from build123d import *

# Parameters (mm, degrees)
SKETCH_2_W          = 58
SKETCH_2_H          = 22
EXTRUDE_1_DEPTH     = 5
SKETCH_4_R          = 10.25
SKETCH_4_R_2        = 1.8
CUT_EXTRUDE_1_DEPTH = 0.5
SKETCH_4_3_R        = 1.8
CUT_EXTRUDE_2_DEPTH = 10
SKETCH_5_W          = 35
SKETCH_5_H          = 4
CUT_EXTRUDE_3_DEPTH = 10
SKETCH_6_R          = 5
CUT_EXTRUDE_4_DEPTH = 3.5
CHAMFER_1_SIZE      = 0.5
CHAMFER_1_SIZE2     = 0.181985117
SKETCH_7_R          = 2
CUT_EXTRUDE_5_DEPTH = 3.5
FILLET_2_R          = 10
FILLET_3_R          = 6
FILLET_4_R          = 20
FILLET_5_R          = 7


with BuildPart() as part:
    # Эскиз2 → Бобышка-Вытянуть1 (new body)
    with BuildSketch(Plane(origin=(0, 0, 0), x_dir=(1, 0, 0), z_dir=(0, 1, 0))):
        Rectangle(SKETCH_2_W, SKETCH_2_H)
    extrude(amount=EXTRUDE_1_DEPTH)

    # Эскиз4 → Вырез-Вытянуть1 (cut)
    with BuildSketch(Plane(origin=(0, 5, 0), x_dir=(1, 0, 0), z_dir=(0, 1, 0))):
        with Locations(Location((-18, 0, 0), (0, 0, 270))):
            Circle(SKETCH_4_R)
        with Locations(Location((-18, 7, 0), (0, 0, 270))):
            Circle(SKETCH_4_R_2, mode=Mode.SUBTRACT)
        with Locations(Location((-18, -7, 0), (0, 0, 270))):
            Circle(SKETCH_4_R_2, mode=Mode.SUBTRACT)
        with Locations(Location((-25, 0, 0), (0, 0, 270))):
            Circle(SKETCH_4_R_2, mode=Mode.SUBTRACT)
        with Locations(Location((-11, 0, 0), (0, 0, 270))):
            Circle(SKETCH_4_R_2, mode=Mode.SUBTRACT)
        with Locations(Location((-18, 0, 0), (0, 0, 270))):
            Circle(SKETCH_4_R_2, mode=Mode.SUBTRACT)
    extrude(amount=-CUT_EXTRUDE_1_DEPTH, mode=Mode.SUBTRACT)

    # Эскиз4<3> → Вырез-Вытянуть2 (cut)
    with BuildSketch(Plane(origin=(0, 5, 0), x_dir=(1, 0, 0), z_dir=(0, 1, 0))):
        with Locations(Location((-18, 7, 0), (0, 0, 270))):
            Circle(SKETCH_4_3_R)
        with Locations(Location((-11, 0, 0), (0, 0, 270))):
            Circle(SKETCH_4_3_R)
        with Locations(Location((-18, -7, 0), (0, 0, 270))):
            Circle(SKETCH_4_3_R)
        with Locations(Location((-25, 0, 0), (0, 0, 270))):
            Circle(SKETCH_4_3_R)
        with Locations(Location((-18, 0, 0), (0, 0, 270))):
            Circle(SKETCH_4_3_R)
    extrude(amount=-CUT_EXTRUDE_2_DEPTH, mode=Mode.SUBTRACT)

    # Эскиз5 → Вырез-Вытянуть3 (cut)
    with BuildSketch(Plane(origin=(0, 5, 0), x_dir=(1, 0, 0), z_dir=(0, 1, 0))):
        with Locations((11.5, 9)):
            Rectangle(SKETCH_5_W, SKETCH_5_H)
        with Locations((11.5, -9)):
            Rectangle(SKETCH_5_W, SKETCH_5_H)
    extrude(amount=-CUT_EXTRUDE_3_DEPTH, mode=Mode.SUBTRACT)

    # Эскиз6 → Вырез-Вытянуть4 (cut)
    with BuildSketch(Plane(origin=(0, 5, 0), x_dir=(1, 0, 0), z_dir=(0, 1, 0))):
        with Locations(Location((22, 0, 0), (0, 0, 270))):
            Circle(SKETCH_6_R)
    extrude(amount=-CUT_EXTRUDE_4_DEPTH, mode=Mode.SUBTRACT)

    # Фаска1
    chamfer_1_edges = [part.edges().sort_by_distance(p)[0] for p in [
        (22, 5, -5),
        (-18, 5, -10.25),
    ]]
    chamfer_1_side = [part.faces().sort_by_distance(p)[0] for p in [
        (1.690967292, 5, 0),
    ]]
    chamfer(chamfer_1_edges, length=CHAMFER_1_SIZE, length2=CHAMFER_1_SIZE2, reference=chamfer_1_side[0])

    # Эскиз7 → Вырез-Вытянуть5 (cut)
    with BuildSketch(Plane(origin=(0, 1.5, 0), x_dir=(1, 0, 0), z_dir=(0, 1, 0))):
        with Locations(Location((22, 0, 0), (0, 0, 270))):
            Circle(SKETCH_7_R)
    extrude(amount=-CUT_EXTRUDE_5_DEPTH, mode=Mode.SUBTRACT)

    # Скругление2
    fillet_2_edges = [part.edges().sort_by_distance(p)[0] for p in [
        (-29, 2.5, 11),
        (-29, 2.5, -11),
    ]]
    fillet(fillet_2_edges, radius=FILLET_2_R)

    # Скругление3
    fillet_3_edges = [part.edges().sort_by_distance(p)[0] for p in [
        (29, 2.5, -7),
        (29, 2.5, 7),
    ]]
    fillet(fillet_3_edges, radius=FILLET_3_R)

    # Скругление4
    # the kernel refuses this fillet: 20 mm, written as the material it takes off along each edge
    with BuildSketch(Plane(origin=(-6, 35, -11), x_dir=(0, 0, 1), z_dir=(0, -1, 0))) as fillet_4_piece_1:
        with BuildLine():
            CenterArc((20, 12), FILLET_4_R, 180, 36.869897646)
            Line((0, 12), (-0.4, 12))
            Line((-0.4, 12), (-0.4, 0))
            Line((-0.4, 0), (0, -0.4))
            ThreePointArc((0, -0.4), (2, -0.4), (3.68, -0.24))
            Line((3.68, -0.24), (4, 0))
        make_face()
    extrude(amount=65, mode=Mode.SUBTRACT)
    with BuildSketch(Plane(origin=(-6, 35, 11), x_dir=(0, 0, -1), z_dir=(0, -1, 0))) as fillet_4_piece_2:
        with BuildLine():
            CenterArc((20, -12), FILLET_4_R, 143.130102354, 36.869897646)
            Line((0, -12), (-0.4, -12))
            Line((-0.4, -12), (-0.4, 0))
            Line((-0.4, 0), (0, 0.4))
            ThreePointArc((0, 0.4), (2, 0.4), (3.68, 0.24))
            Line((3.68, 0.24), (4, 0))
        make_face()
    extrude(amount=65, mode=Mode.SUBTRACT)

    # Скругление5
    fillet_5_edges = [part.edges().sort_by_distance(p)[0] for p in [
        (-6, 2.5, -7),
        (-6, 2.5, 7),
    ]]
    fillet(fillet_5_edges, radius=FILLET_5_R)


solid = part.part
Verification items for the finished model (mm, model axes). A direction names the side the tool comes from. Round coordinates to 2 decimals unless told otherwise and drop trailing zeros. Loops run counter-clockwise (first coordinate to the right, second up) from the corner with the lowest first, then second, coordinate; pieces in that order, holes last. Notation, with made-up numbers: (50.25, 15) - (80.25, 15) arc R14 ccw to (80.25, 19) - close; hole circle Ø2 at (7.25, 6.5). An arc over 180 degrees is marked (long way). Answer in a Markdown table with one row per item. Add a question column.
Q1. Gauge pin test, flat ends, axial feed: pin 1 (9 mm diameter, centred on x = 22, z = 0, fed in from +Y); pin 2 (1.5 mm diameter, centred on x = 7.5, y = 2.5, fed in from -Z); pin 3 (6 mm diameter, centred on x = -16.5, z = 3, fed in from +Y). Record the tip position at first contact, or that the pin passes through.
Q2. Section check B-B on x = 22. Enter the section's corners in (y, z).
Q3. Section check A-A on z = 0. State how many separate pieces and enclosed holes the cut face has, plus the area to 3 significant figures.
Q4. Material ranges on line 1 (X direction, y = 1.75, z = 0); line 2 (X direction, y = 2.8, z = -1.5); line 3 (Y direction, x = -15, z = 7.5), recorded low to high.
Q5. Section check C-C on y = 0.7. Enter the section's corners in (x, z), plus the area to 3 significant figures.
Q6. Tool access check on faces 4 (the face through (-18.5, 2.5, 11)), 5 (the face through (9, 3, -7)), 6 (the face through (17.12, 3.18, -1.08)), 7 (the face through (9, 3, 7)). Record the directions out of +Z, -Z, +X, -X, +Y, -Y that give a thin tool (end or side, any length) a straight path to the whole face; none if there is none.
Q7. Release check for a two-part mould opening along Z. For faces 1 (the face through (-18.5, 2.5, -11)), 2 (the face through (-5.737, 2.465, 7.257)), 3 (the face through (-18, 4.5, 2)) record: pulls with the +Z half, pulls with the -Z half, needs draft (parallel to the pull), parting line crosses it, or undercut.
Q8. Section check D-D on x = 4.5. Enter the section's corners in (y, z).
Found:
| question | item | result |
|---|---|---|
| 1 | pin 1 | stops at y = 1.5 |
| 1 | pin 2 | stops at z = -7 |
| 1 | pin 3 | stops at y = 4.5 |
| 2 | outline | (0, -7) - (5, -7) - (5, -5.5) - (4.82, -5) - (1.5, -5) - (1.5, -2) - (0, -2) - close; (0, 2) - (1.5, 2) - (1.5, 5) - (4.82, 5) - (5, 5.5) - (5, 7) - (0, 7) - close |
| 3 | separate pieces | 5 |
| 3 | enclosed holes | 0 |
| 3 | area | 190 mm² |
| 4 | line 1 | x = -29 to -26.8, -23.2 to -19.8, -16.2 to -12.8, -9.2 to 17, 27 to 29 |
| 4 | line 2 | x = -28.99 to -25.99, -24.01 to -18.99, -17.01 to -11.99, -10.01 to 17.23, 26.77 to 28.98 |
| 4 | line 3 | y = 0 to 4.5 |
| 5 | outline | (-29, -1) arc R10 ccw to (-19, -11) - (-18, -11) arc R20 ccw to (-7.52, -8.04) arc R7 cw to (-3.86, -7) - (23, -7) arc R6 ccw to (29, -1) - (29, 1) arc R6 ccw to (23, 7) - (-3.86, 7) arc R7 cw to (-7.52, 8.04) arc R20 ccw to (-18, 11) - (-19, 11) arc R10 ccw to (-29, 1) - close; hole circle Ø3.6 at (-25, 0); hole circle Ø3.6 at (-18, -7); hole circle Ø3.6 at (-18, 0); hole circle Ø3.6 at (-18, 7); hole circle Ø3.6 at (-11, 0); hole circle Ø4 at (22, 0) |
| 5 | area | 844 mm² |
| 6 | face 4 | +Z, +X, -X, +Y, -Y |
| 6 | face 5 | -Z, +X, +Y, -Y |
| 6 | face 6 | +Y |
| 6 | face 7 | +Z, +X, +Y, -Y |
| 7 | face 1 | pulls with the -Z half |
| 7 | face 2 | pulls with the +Z half |
| 7 | face 3 | undercut |
| 8 | outline | (0, -7) - (5, -7) - (5, 7) - (0, 7) - close |
